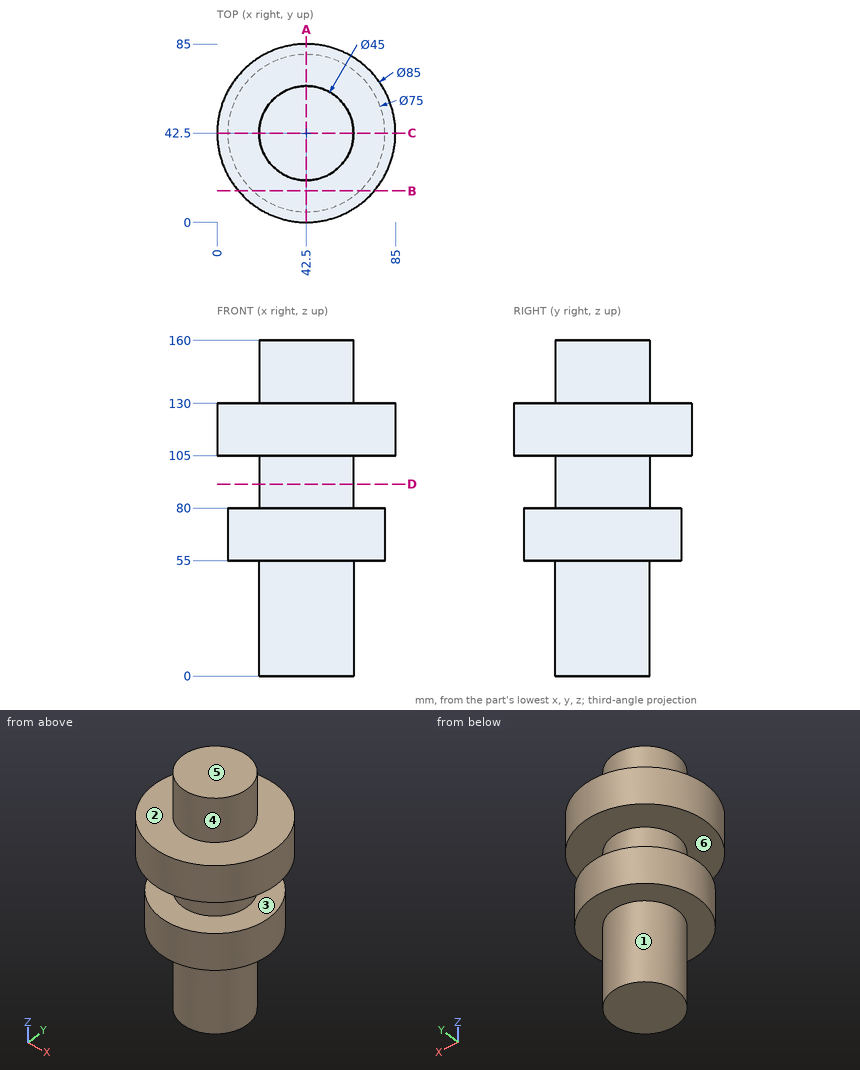
Geometry check sheet. Reference: drawing and pictorial views, mm from the part's lowest x, y, z. A direction names the side the tool comes from. Give positions to 0.01 mm unless a question says otherwise; leave off trailing zeros. Order: outer loops, then holes, each group sorted by start corner. A loop starts at its lowest first (then second) coordinate and runs counter-clockwise, first axis right, second up. Notation, with made-up numbers: (61.25, -12.5) -> (67.25, -12.5) arc R24 ccw to (67.25, 21.5) -> close; hole circle Ø8 at (15.25, -20.75). An arc over 180 degrees is marked (long way). Use CSV: the item, a comma, the result in double quotes. Start each with the question number.
1) Mould release check, pull along Z, two halves, no side actions. Record for the marked faces 4, 5 and 6: released by +Z, released by -Z, zero draft, split by the parting line, or undercut.
2) Go/stop test with flat-tipped pins: P1, Ø10, axis at x = 66.5, y = 72.5, coming from the -Z side; P2, Ø3, axis at x = 65.5, y = 64, coming from the +Z side; P3, Ø5, axis at y = 64.5, z = 113.5, coming from the +X side. Record where each tip stops, or that it passes through.
3) Material ranges on line 1 (Z direction, x = 33, y = 70.5); line 2 (Z direction, x = 63, y = 77); line 3 (X direction, y = 44, z = 63), recorded low to high. Write a range as from..to.
4) Sectioned sample at D-D, the plane z = 91.5. Record the boundary of the cut face in (x, y).
5) Sectioned sample at A-A, the plane x = 42.5. Record the boundary of the cut face in (y, z).
6) Sectioned sample at B-B, the plane y = 15. Record the boundary of the cut face in (x, z), plus the area to 3 significant figures.
7) Set-up check for the marked faces 1, 2 and 3: record each of +Z, -Z, +X, -X, +Y, -Y from which the full face is reachable in a straight line by a thin tool's end or side.
Recorded:
1,face 4,"zero draft"
1,face 5,"released by +Z"
1,face 6,"undercut"
2,P1,"z = 55"
2,P2,"z = 130"
2,P3,"x = 80.26"
3,line 1,"55..80, 105..130"
3,line 2,"105..130"
3,line 3,"5.03..79.97"
4,outline,"circle Ø45 at (42.5, 42.5)"
5,outline,"(0, 105) -> (20, 105) -> (20, 80) -> (5, 80) -> (5, 55) -> (20, 55) -> (20, 0) -> (65, 0) -> (65, 55) -> (80, 55) -> (80, 80) -> (65, 80) -> (65, 105) -> (85, 105) -> (85, 130) -> (65, 130) -> (65, 160) -> (20, 160) -> (20, 130) -> (0, 130) -> close"
6,outline,"(10.1, 105) -> (74.9, 105) -> (74.9, 130) -> (10.1, 130) -> close; (17, 55) -> (68, 55) -> (68, 80) -> (17, 80) -> close"
6,area,"2,890 mm2"
7,face 1,"-Z"
7,face 2,"+Z"
7,face 3,"none"
